Could you check a few things on this drawing? It's one solid part, dimensions in mm from its lowest x, y, z. Coordinates: 2 decimals unless noted, no trailing zeros. Order: outer loops, then holes, each group sorted by start corner. A loop starts at its lowest first (then second) coordinate and runs counter-clockwise, first axis right, second up. Notation, with made-up numbers: (60, 59.5) -> (91, 59.5) arc R24 ccw to (91, 89.5) -> close; hole circle Ø5 at (45, 1.25). An arc over 180 degrees is marked (long way). Use a Markdown table: item, result. Add a question column.
1. If I drill on line 1 along Z through (x, y) = (1.5, 1.55); line 2 along X through (y, z) = (1, 37), over which ranges is the centre line in solid material (lowest first)? Write a range as from..to.
2. For pin 1 Ø1.5 at (x, y) = (1, 2) entering from +Z; pin 2 Ø0.9 at (x, y) = (1, 1) entering from -Z; pin 3 Ø0.9 at (y, z) = (1.5, 138.5) entering from +X, each with a flat end and sliding along its axis, tell me the tip position at first contact or that it passes through.
3. Suppose I cut it at B-B, the plane x = 119.5. List the corners of the cut face in (y, z) for me.
4. Suppose I cut it at A-A, the plane y = 2.1. State how many separate pieces and enclosed holes the cut face has, then the cut area to 3 significant figures.
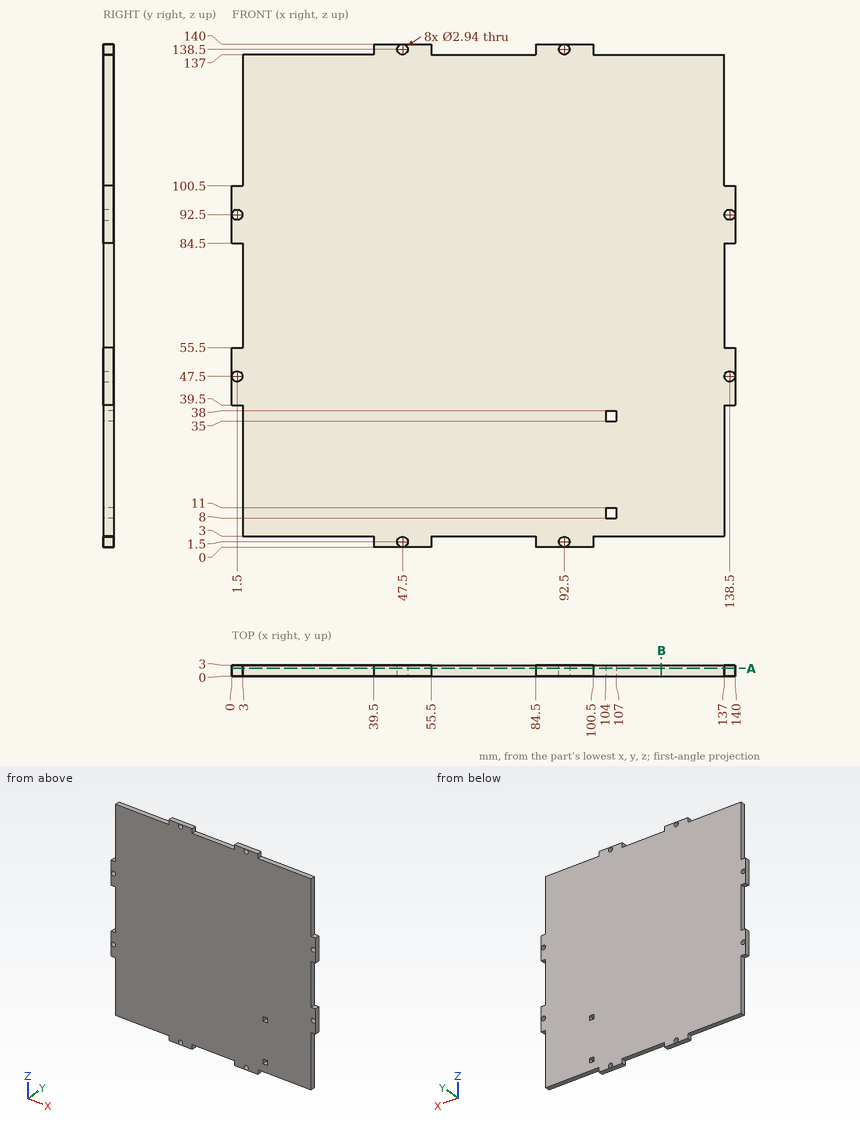
Worked out:
| question | item | result |
|---|---|---|
| 1 | line 1 | z = 39.5..46.03, 48.97..55.5, 84.5..91.03, 93.97..100.5 |
| 1 | line 2 | x = 3..104, 107..137 |
| 2 | pin 1 | stops at z = 100.5 |
| 2 | pin 2 | stops at z = 39.5 |
| 2 | pin 3 | stops at x = 100.5 |
| 3 | outline | (0, 3) -> (3, 3) -> (3, 137) -> (0, 137) -> close |
| 4 | separate pieces | 1 |
| 4 | enclosed holes | 10 |
| 4 | area | 18,300 mm² |
